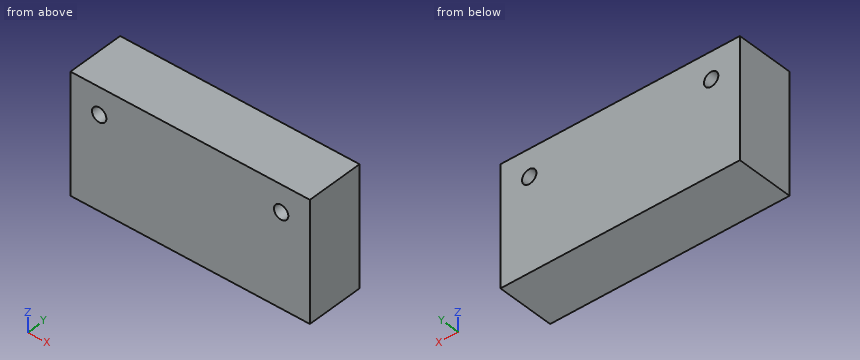
```python
from build123d import *

# Parameters (mm, degrees)
SKETCH1_W           = 50
SKETCH1_H           = 12
BOSS_EXTRUDE1_DEPTH = 25
CUT_EXTRUDE1_REACH  = 39.336
SKETCH2_R           = 1.5


with BuildPart() as part:
    # Sketch1 → Boss-Extrude1 (new body)
    with BuildSketch(Plane.XY):
        Rectangle(SKETCH1_W, SKETCH1_H)
    extrude(amount=BOSS_EXTRUDE1_DEPTH)

    # Sketch2 → Cut-Extrude1 (cut, up to next)
    with BuildSketch(Plane.XZ.offset(6), mode=Mode.PRIVATE) as cut_extrude1_sk1:
        with Locations(Location((-19, 19.395863619, 0), (0, 0, 270))):
            Circle(SKETCH2_R)
    cut_extrude1_tool1 = extrude(cut_extrude1_sk1.sketch, amount=-CUT_EXTRUDE1_REACH, mode=Mode.PRIVATE) & part.part
    # Sketch2 → Cut-Extrude1 (cut, up to next)
    with BuildSketch(Plane.XZ.offset(6), mode=Mode.PRIVATE) as cut_extrude1_sk2:
        with Locations(Location((19, 19.395863619, 0), (0, 0, 270))):
            Circle(SKETCH2_R)
    cut_extrude1_tool2 = extrude(cut_extrude1_sk2.sketch, amount=-CUT_EXTRUDE1_REACH, mode=Mode.PRIVATE) & part.part
    add(cut_extrude1_tool1.solids().sort_by_distance((-19, -6, 19.395864))[0], mode=Mode.SUBTRACT)
    add(cut_extrude1_tool2.solids().sort_by_distance((19, -6, 19.395864))[0], mode=Mode.SUBTRACT)


solid = part.part
```
Here's how the part is built. I have some questions about the finished solid (model axes, mm). Coordinates: 2 decimals unless noted, no trailing zeros. Loops run counter-clockwise (first coordinate to the right, second up) from the corner with the lowest first, then second, coordinate; pieces in that order, holes last. Notation, with made-up numbers: (64.25, -36.75) -> (121.25, -36.75) arc R21 cw to (121.25, -26.75) -> close; hole circle Ø9 at (-35, -10). An arc over 180 degrees is marked (long way). Return JSON: item names as keys, results as strings.
1) I need wall thicknesses on line 1 (X direction, y = 3.75, z = 18.5). Which ranges of the line are inside material? Lowest first, please. Write a range as from..to.
Results below:
{"line 1": "-25..-20.2, -17.8..17.8, 20.2..25"}
2) If we section it at A-A, the plane x = -19: Write out the boundary of the cut face in (y, z).
Results below:
{"outline": "(-6, 0) -> (6, 0) -> (6, 17.9) -> (-6, 17.9) -> close; (-6, 20.9) -> (6, 20.9) -> (6, 25) -> (-6, 25) -> close"}
3) If we section it at B-B, the plane z = 18.5: Write out the boundary of the cut face in (x, y), then the cut area to 3 significant figures.
Results below:
{"outline": "(-25, -6) -> (-20.2, -6) -> (-20.2, 6) -> (-25, 6) -> close; (-17.8, -6) -> (17.8, -6) -> (17.8, 6) -> (-17.8, 6) -> close; (20.2, -6) -> (25, -6) -> (25, 6) -> (20.2, 6) -> close", "area": "542 mm²"}
4) Will these pins go through, and if not, where does the flat tip stop? pin 1 (1.5 mm diameter, centred on x = -12.5, y = 1, fed in from -Z); pin 2 (2.5 mm diameter, centred on x = 19, z = 19.4, fed in from +Y).
Results below:
{"pin 1": "z = 0", "pin 2": "through"}
